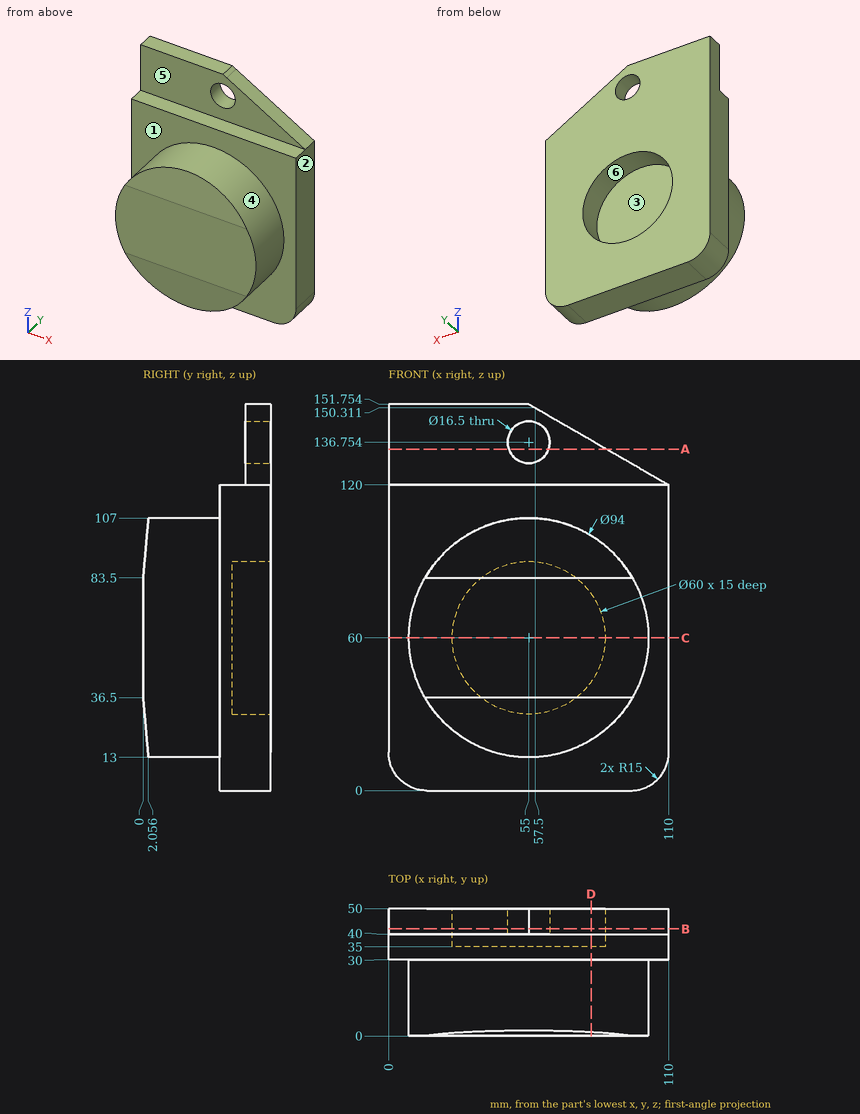
For this review, use the dimensioned drawing (mm, ordinates from the lowest corner) and the shaded views. A direction names the side the tool comes from. Round coordinates to 2 decimals unless told otherwise and drop trailing zeros. Write each loop counter-clockwise with the first axis right and the second up, starting at its lowest first coordinate (ties: lowest second). Pieces come first, ordered by that corner, then holes. Notation, with made-up numbers: (47, 81) -> (70, 81) arc R29 ccw to (70, 119) -> close; hole circle Ø2 at (-15.75, 72.5). An arc over 180 degrees is marked (long way). Use one line per item in the form item = value.
Q1. To check wall thickness, follow probe 1 along Z at (x, y) = (55, 43.25) (1 decimal); probe 2 along X at (y, z) = (40, 60); probe 3 along Z at (x, y) = (55, 39.25). State the ranges of each line that lie inside material, in increasing order. Write a range as from..to.
Resolved:
probe_1 = 0..30, 90..128.5, 145..151.8
probe_2 = 0..25, 85..110
probe_3 = 0..30, 90..120
Q2. Clearance check with flat-ended pins moving along their axes: pin 1 Ø8 at (x, z) = (12.5, 116) entering from -Y; pin 2 Ø2 at (x, y) = (42.5, 17.5) entering from -Z; pin 3 Ø6 at (y, z) = (16.5, 36.5) entering from +X. State where each tip first meets the part, or that it passes through.
Resolved:
pin_1 = 30
pin_2 = 14.43
pin_3 = 97.29
Q3. Machinability: for the marked faces 4, 5 and 6, which of the approach directions +Z, -Z, +X, -X, +Y, -Y give a long, thin tool a straight path to every point of the face, cutting with its end or side? Answer none if there is none.
Resolved:
face_4 = -Y
face_5 = +Z, +X, -X, -Y
face_6 = +Y
Q4. Consider section C-C (z = 60). State the section outline as (x, y) points, then the cut area to 3 significant figures.
Resolved:
outline = (0, 30) -> (8, 30) -> (8, 0) -> (102, 0) -> (102, 30) -> (110, 30) -> (110, 50) -> (85, 50) -> (85, 35) -> (25, 35) -> (25, 50) -> (0, 50) -> close
area = 4,120 mm²
Q5. The part is to be moulded in two halves that separate along X. For the marked faces 1, 2 and 3, say which applies: released by +X, released by -X, zero draft, split by the parting line, or undercut.
Resolved:
face_1 = zero draft
face_2 = released by +X
face_3 = undercut
Q6. Consider section D-D (x = 79.5). State the section outline as (y, z) points, then the cut area to 3 significant figures.
Resolved:
outline = (0, 36.5) -> (1.45, 19.89) -> (30, 19.89) -> (30, 0) -> (50, 0) -> (50, 42.69) -> (35, 42.69) -> (35, 77.31) -> (50, 77.31) -> (50, 137.61) -> (40, 137.61) -> (40, 120) -> (30, 120) -> (30, 100.11) -> (1.45, 100.11) -> (0, 83.5) -> close
area = 4,440 mm²
Q7. Consider section A-A (z = 134). State the section outline as (x, y) points, then the cut area to 3 significant figures.
Resolved:
outline = (0, 40) -> (47.22, 40) -> (47.22, 50) -> (0, 50) -> close; (62.78, 40) -> (85.75, 40) -> (85.75, 50) -> (62.78, 50) -> close
area = 702 mm²
Q8. Consider section B-B (y = 42). State the section outline as (x, z) points.
Resolved:
outline = (0, 15) arc R15 ccw to (15, 0) -> (95, 0) arc R15 ccw to (110, 15) -> (110, 120) -> (57.5, 150.31) -> (55, 151.75) -> (0, 151.75) -> close; hole circle Ø60 at (55, 60); hole circle Ø16.5 at (55, 136.75)
